from build123d import *

# Parameters (mm, degrees)
SKETCH2_R           = 25
SKETCH2_R_2         = 2.5
BOSS_EXTRUDE1_DEPTH = 3
SKETCH3_R           = 8
SKETCH3_R_2         = 4
BOSS_EXTRUDE2_DEPTH = 10


with BuildPart() as part:
    # Sketch2 → Boss-Extrude1 (new body)
    with BuildSketch(Plane(origin=(0, 0, 0), x_dir=(1, 0, 0), z_dir=(0, 1, 0))):
        Circle(SKETCH2_R)
        with Locations((-18.5, 0)):
            Circle(SKETCH2_R_2, mode=Mode.SUBTRACT)
        with Locations((0, 18.5)):
            Circle(SKETCH2_R_2, mode=Mode.SUBTRACT)
        with Locations((18.5, 0)):
            Circle(SKETCH2_R_2, mode=Mode.SUBTRACT)
        with Locations((0, -18.5)):
            Circle(SKETCH2_R_2, mode=Mode.SUBTRACT)
    extrude(amount=BOSS_EXTRUDE1_DEPTH)

    # Sketch3 → Boss-Extrude2 (add)
    with BuildSketch(Plane(origin=(0, 3, 0), x_dir=(1, 0, 0), z_dir=(0, 1, 0))):
        Circle(SKETCH3_R)
        Circle(SKETCH3_R_2, mode=Mode.SUBTRACT)
    extrude(amount=BOSS_EXTRUDE2_DEPTH)


solid = part.part
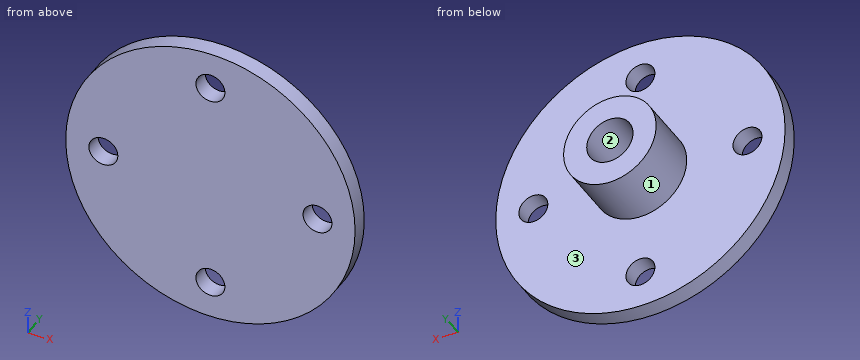
Input: part model. Units: mm. Frame: model coordinates. Face numbers are marked on the shaded views. Coordinates: 2 decimals unless noted, no trailing zeros. Order: outer loops, then holes, each group sorted by start corner. A loop starts at its lowest first (then second) coordinate and runs counter-clockwise, first axis right, second up. Notation, with made-up numbers: M -30,-24 L 24,-24 A22 ccw 24,13 Z; hole C -25.75,59.5 d9. An arc over 180 degrees is marked long. Answer in a Markdown table with one row per item.
(1) Material intervals for line 1 (Z direction, x = 0, y = 1.6); line 2 (Z direction, x = 0, y = 6.5), sorted ascending. Write a range as [from, to].
Numbers:
| item | result |
|---|---|
| line 1 | z = [-25, -21], [-16, 16], [21, 25] |
| line 2 | z = [-8, -4], [4, 8] |
(2) Section query B-B, the plane x = 0. Output: boundary loops of the cut face in (y, z).
Numbers:
| item | result |
|---|---|
| outline | M 0,-25 L 3,-25 L 3,-21 L 0,-21 Z; M 0,-16 L 3,-16 L 3,-8 L 13,-8 L 13,-4 L 3,-4 L 3,4 L 13,4 L 13,8 L 3,8 L 3,16 L 0,16 Z; M 0,21 L 3,21 L 3,25 L 0,25 Z |
(3) Draft query along X for the marked faces 1, 2 and 3. Return one class per face: pulls with the +X half, pulls with the -X half, needs draft (parallel to the pull), parting line crosses it, or undercut.
Numbers:
| item | result |
|---|---|
| face 1 | parting line crosses it |
| face 2 | undercut |
| face 3 | needs draft |
(4) Section query D-D, the plane z = 17. Output: boundary loops of the cut face in (x, y).
Numbers:
| item | result |
|---|---|
| outline | M -18.33,0 L -2,0 L -2,3 L -18.33,3 Z; M 2,0 L 18.33,0 L 18.33,3 L 2,3 Z |
(5) Contact query for flat-ended pins moving along their axis: pin 1 Ø2.5 at (x, z) = (-2, -0.5) entering from +Y; pin 2 Ø2 at (x, y) = (-14, 5) entering from +Z; pin 3 Ø4 at (x, y) = (15.5, 4) entering from +Z; pin 4 Ø5 at (y, z) = (3, -17) entering from +X. Output: stop coordinate, or through.
Numbers:
| item | result |
|---|---|
| pin 1 | stops at y = 3 |
| pin 2 | passes through |
| pin 3 | stops at z = 20.87 |
| pin 4 | stops at x = 20.37 |
(6) Section query C-C, the plane y = 1.5. Output: boundary loops of the cut face in (x, z).
Numbers:
| item | result |
|---|---|
| outline | C 0,0 d50; hole C -18.5,0 d5; hole C 0,-18.5 d5; hole C 0,18.5 d5; hole C 18.5,0 d5 |
(7) Section query A-A, the plane z = 0. Output: boundary loops of the cut face in (x, y).
Numbers:
| item | result |
|---|---|
| outline | M -25,0 L -21,0 L -21,3 L -25,3 Z; M -16,0 L 16,0 L 16,3 L 8,3 L 8,13 L 4,13 L 4,3 L -4,3 L -4,13 L -8,13 L -8,3 L -16,3 Z; M 21,0 L 25,0 L 25,3 L 21,3 Z |
